```python
from build123d import *

# Parameters (mm, degrees)
F2_DEPTH = 14
F3_DEPTH = 14.001


with BuildPart() as f2:
    # F0 (on Top) → F2 (new body)
    with BuildSketch(Plane.XY):
        with BuildLine():
            Line((0, 11), (-22, 4))
            ThreePointArc((-22, 4), (-26, 0), (-22, -4))
            Line((-22, -4), (0, -11))
            ThreePointArc((0, -11), (11, 0), (0, 11))
        make_face()
    extrude(amount=F2_DEPTH)

    # F1 (on face) → F3 (cut, through all)
    with BuildSketch(Plane.XY):
        with BuildLine():
            ThreePointArc((-21.862283, 3.046889), (-25.05, 0), (-21.862283, -3.046889))
            Line((-21.862283, -3.046889), (0.14424, -10.048965))
            ThreePointArc((0.14424, -10.048965), (10.05, 0), (0.14424, 10.048965))
            Line((0.14424, 10.048965), (-21.862283, 3.046889))
        make_face()
    extrude(amount=F3_DEPTH, mode=Mode.SUBTRACT)


solid = f2.part
```
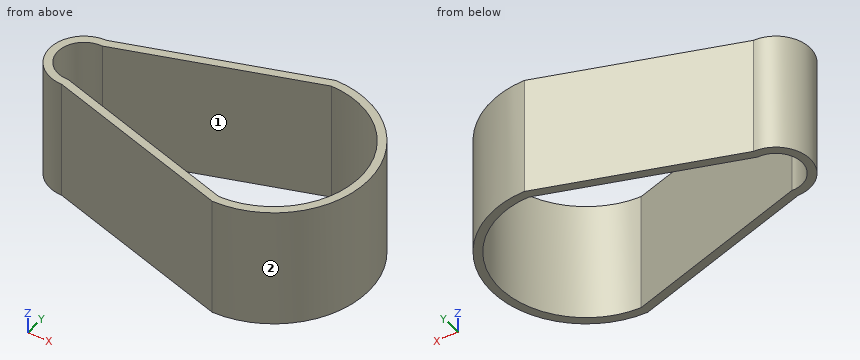
Read the model definition and answer for the solid it produces. Units are mm, in the model's axes. Face numbers are marked on the shaded views. A direction names the side the tool comes from. Coordinates: 2 decimals unless noted, no trailing zeros. Write each loop counter-clockwise with the first axis right and the second up, starting at its lowest first coordinate (ties: lowest second). Pieces come first, ordered by that corner, then holes. Notation, with made-up numbers: (-4, 27.25) - (19, 27.25) arc R36 cw to (19, 64.25) - close; hole circle Ø2 at (28, -39.75). An arc over 180 degrees is marked (long way). Answer as a JSON object with one key per item and string values. Group by question number.
1. Consider L1, parallel to X at y = -1.75, z = 2.25; L2, parallel to Y at x = 5.5, z = 5.75; L3, parallel to Y at x = -7.5, z = 8.25. Determine where each line is inside the solid, lowest interval first. Write a range as [from, to].
2. Which of the six approach directions +Z, -Z, +X, -X, +Y, -Y give full straight-line access (tool end or side, diameter ignored) to the marked faces 1 and 2?
3. Each of these flat-tipped pins is pushed along its axis until it touches: P1, Ø3, axis at x = -4, z = 2.5, coming from the -Y side; P2, Ø5, axis at y = 5.5, z = 9.5, coming from the +X side; P3, Ø1, axis at y = -1, z = 6.5, coming from the +X side. Where does it stop, or does it pass through?
4. A cutting plane is placed at A-A (z = 1.5). Determine the outline of the cut face in (x, y).
5. A cutting plane is placed at B-B (y = 0). Determine the outline of the cut face in (x, z), plus the area to 3 significant figures.
6. A cutting plane is placed at C-C (x = -12.5). Determine the outline of the cut face in (y, z).
Worked out:
{
 "1": {"L1": "x = [-25.6, -24.5], [9.9, 10.86]", "L2": "y = [-9.53, -8.41], [8.41, 9.53]", "L3": "y = [-8.61, -7.62], [7.62, 8.61]"},
 "2": {"face 1": "+Z, -Z", "face 2": "+Z, -Z, +X"},
 "3": {"P1": "stops at y = -10.2", "P2": "stops at x = 10.58", "P3": "stops at x = 10.99"},
 "4": {"outline": "(-22, -4) - (0, -11) arc R11 ccw to (0, 11) - (-22, 4) arc R4 ccw to start; hole (-21.86, -3.05) - (0.14, -10.05) arc R10.05 ccw to (0.14, 10.05) - (-21.86, 3.05) arc R3.05 ccw (long way) to start"},
 "5": {"outline": "(-26, 0) - (-25.05, 0) - (-25.05, 14) - (-26, 14) - close; (10.05, 0) - (11, 0) - (11, 14) - (10.05, 14) - close", "area": "26.6 mm²"},
 "6": {"outline": "(-7.02, 0) - (-6.03, 0) - (-6.03, 14) - (-7.02, 14) - close; (6.03, 0) - (7.02, 0) - (7.02, 14) - (6.03, 14) - close"}
}
